from build123d import *

# Parameters (mm, degrees)
EXTRUSION1_DEPTH = 5
EXTRUSION2_REACH = 109.744


with BuildPart() as part:
    # Esquisse1 → Extrusion1 (new body)
    with BuildSketch(Plane.XY):
        Polygon((-48.749448329, -48.162307692), (-34.749448329, -48.162307692), (-34.749448329, -23.162307692), (25.250551671, -23.162307692), (25.250551671, -48.162307692), (96.250551671, -48.162307692), (96.250551671, 2.837692308), (-48.749448329, 2.837692308), align=None)
    extrude(amount=EXTRUSION1_DEPTH)

    # Esquisse3 → Extrusion2 (cut, up to next)
    with BuildSketch(Plane(origin=(0, 0, 0), x_dir=(-1, 0, 0), z_dir=(0, 0, -1)), mode=Mode.PRIVATE) as extrusion2_sk1:
        with BuildLine():
            Line((-25.250551671, -23.162307692), (-65.250551671, -23.162307692))
            ThreePointArc((-65.250551671, -23.162307692), (-72.321619482, -26.09123988), (-75.250551671, -33.162307692))
            Line((-75.250551671, -33.162307692), (-75.250551671, -48.162307692))
            Line((-75.250551671, -48.162307692), (-25.250551671, -48.162307692))
            Line((-25.250551671, -48.162307692), (-25.250551671, -23.162307692))
        make_face()
    extrusion2_tool1 = extrude(extrusion2_sk1.sketch, amount=-EXTRUSION2_REACH, mode=Mode.PRIVATE) & part.part
    add(extrusion2_tool1.solids().sort_by_distance((49.852869, -35.84164, 0))[0], mode=Mode.SUBTRACT)


solid = part.part
Geometry: final body of the model. Coordinates: model frame, mm. A direction names the side the tool comes from. Round coordinates to 2 decimals unless told otherwise and drop trailing zeros. Loops run counter-clockwise (first coordinate to the right, second up) from the corner with the lowest first, then second, coordinate; pieces in that order, holes last. Notation, with made-up numbers: (79.25, -23) - (135.25, -23) arc R8 cw to (135.25, -9) - close; hole circle Ø3 at (45.5, 56.25). An arc over 180 degrees is marked (long way). Write each question's results on one line, items separated by ' | '. Start each with the question number.
1) Cut plane D-D on y = -26. Return loops of the section in (x, z).
2) Cut plane C-C on x = 32. Return loops of the section in (y, z), then the cut area to 3 significant figures.
3) Cut plane B-B on y = -34.5. Return loops of the section in (x, z), then the cut area to 3 significant figures.
4) First-contact query: P1, Ø2, axis at x = 5, z = 4.5, coming from the -Y side; P2, Ø2, axis at x = -12, y = -7, coming from the -Z side. Flat tips, straight axial feed; report the tip coordinate or a pass-through.
5) Access query for faces 1 (the face through (96.251, -23, 2)), 2 (the face through (15, -23.162, 2)). Directions: +Z, -Z, +X, -X, +Y, -Y. A direction counts if a zero-diameter tool reaches every point of the face in a straight line with its end or side. Return the directions, or none.
6) Cut plane A-A on z = 0.8. Return loops of the section in (x, y), then the cut area to 3 significant figures.
7) Line query: probe 1 along X at (y, z) = (-37, 0.9); probe 2 along Y at (x, z) = (1, 2.7); probe 3 along X at (y, z) = (-32.5, 3.2). Output: solid intervals per line, ascending. Write a range as [from, to].
Verdict:
1) outline: (-48.75, 0) - (-34.75, 0) - (-34.75, 5) - (-48.75, 5) - close; (72.23, 0) - (96.25, 0) - (96.25, 5) - (72.23, 5) - close
2) outline: (-23.16, 0) - (2.84, 0) - (2.84, 5) - (-23.16, 5) - close | area: 130 mm2
3) outline: (-48.75, 0) - (-34.75, 0) - (-34.75, 5) - (-48.75, 5) - close; (75.25, 0) - (96.25, 0) - (96.25, 5) - (75.25, 5) - close | area: 175 mm2
4) P1: stops at y = -23.16 | P2: stops at z = 0
5) face 1: +Z, -Z, +X, +Y, -Y | face 2: +Z, -Z, -Y
6) outline: (-48.75, -48.16) - (-34.75, -48.16) - (-34.75, -23.16) - (65.25, -23.16) arc R10 cw to (75.25, -33.16) - (75.25, -48.16) - (96.25, -48.16) - (96.25, 2.84) - (-48.75, 2.84) - close | area: 4,670 mm2
7) probe 1: x = [-48.75, -34.75], [75.25, 96.25] | probe 2: y = [-23.16, 2.84] | probe 3: x = [-48.75, -34.75], [75.23, 96.25]
